```python
from build123d import *

# Parameters (mm, degrees)
BOSS_EXTRUDE1_DEPTH     = 2
SCALE1_SCALE            = 2
SKETCH6_R               = 1.5
CUT_EXTRUDE2_DEPTH      = 50.464206186
SKETCH7_W               = 25
SKETCH7_H               = 3
BOSS_EXTRUDE2_DEPTH     = 15
SKETCH8_R               = 1.5
SKETCH8_W               = 16
SKETCH8_H               = 11
CUT_EXTRUDE3_DEPTH      = 18
FILLET3_R               = 3
FILLET4_R               = 3
SKETCH10_R              = 1.5
CUT_EXTRUDE4_DEPTH      = 10
CUT_EXTRUDE5_DEPTH      = 52.533558907
CUT_EXTRUDE5_DEPTH_BACK = 52.533558907
SKETCH11_W              = 25
SKETCH11_H              = 3
CUT_EXTRUDE6_DEPTH      = 50.464206186
CUT_EXTRUDE6_DEPTH_BACK = 50.464206186


with BuildPart() as part:
    # Sketch2 → Boss-Extrude1 (new body)
    with BuildSketch(Plane(origin=(0, 0, 0), x_dir=(1, 0, 0), z_dir=(0, 1, 0))):
        with BuildLine():
            Line((-17.967387551, 9.159795774), (-20.639475337, 7.15016677))
            ThreePointArc((-20.639475337, 7.15016677), (-18.649238809, 4.17439457), (-19.346117765, 0.662896123))
            ThreePointArc((-19.346117765, 0.662896123), (-19.45411943, -1.286546543), (-18.558961711, -3.021678736))
            ThreePointArc((-18.558961711, -3.021678736), (-16.421478173, -5.190969631), (-13.78312899, -6.712078584))
            ThreePointArc((-13.78312899, -6.712078584), (-13.032173848, -6.916004841), (-12.276686285, -7.102440046))
            ThreePointArc((-12.276686285, -7.102440046), (-12.194265553, -8.245293076), (-11.737308023, -9.296052821))
            ThreePointArc((-11.737308023, -9.296052821), (-10.975506649, -9.937799505), (-10.090124565, -10.394175126))
            Line((-10.090124565, -10.394175126), (-7.391598262, -11.698651137))
            Line((-7.391598262, -11.698651137), (7.391598262, -11.698651137))
            Line((7.391598262, -11.698651137), (10.090124565, -10.394175126))
            ThreePointArc((10.090124565, -10.394175126), (10.975506649, -9.937799505), (11.737308023, -9.296052821))
            ThreePointArc((11.737308023, -9.296052821), (12.194265553, -8.245293076), (12.276686285, -7.102440046))
            ThreePointArc((12.276686285, -7.102440046), (13.032173848, -6.916004841), (13.78312899, -6.712078584))
            ThreePointArc((13.78312899, -6.712078584), (16.421478173, -5.190969631), (18.558961711, -3.021678736))
            ThreePointArc((18.558961711, -3.021678736), (19.45411943, -1.286546543), (19.346117765, 0.662896123))
            ThreePointArc((19.346117765, 0.662896123), (18.649238809, 4.17439457), (20.639475337, 7.15016677))
            Line((20.639475337, 7.15016677), (17.967387551, 9.159795774))
            ThreePointArc((17.967387551, 9.159795774), (10.858325227, 7.499674132), (4.169484372, 10.424426945))
            Line((4.169484372, 10.424426945), (2.224138848, 10.424426945))
            Line((2.224138848, 10.424426945), (0.696104526, 13.114793475))
            Line((0.696104526, 13.114793475), (0, 13.358013588))
            Line((0, 13.358013588), (-0.696104526, 13.114793475))
            Line((-0.696104526, 13.114793475), (-2.224138848, 10.424426945))
            Line((-2.224138848, 10.424426945), (-4.169484372, 10.424426945))
            ThreePointArc((-4.169484372, 10.424426945), (-10.858325227, 7.499674132), (-17.967387551, 9.159795774))
        make_face()
    extrude(amount=BOSS_EXTRUDE1_DEPTH)


with BuildPart() as part_1:
    # Scale1: scaled about (0, 1, 0.242383844)
    add(part.part.scale(SCALE1_SCALE).moved(Location((0, -1, -0.242383844))))

    # Sketch6 → Cut-Extrude2 (cut, through all)
    with BuildSketch(Plane(origin=(0, 3, 0), x_dir=(1, 0, 0), z_dir=(0, 1, 0))):
        with Locations(Location((-5.851533015, 16.28357055, 0), (0, 0, 270))):
            Circle(SKETCH6_R)
        with Locations(Location((4.151829214, 16.28357055, 0), (0, 0, 270))):
            Circle(SKETCH6_R)
    extrude(amount=-CUT_EXTRUDE2_DEPTH, mode=Mode.SUBTRACT)

    # Sketch7 → Boss-Extrude2 (add)
    with BuildSketch(Plane(origin=(0, 3, 0), x_dir=(1, 0, 0), z_dir=(0, 1, 0))):
        with Locations((0, 11.610861671)):
            Rectangle(SKETCH7_W, SKETCH7_H)
    extrude(amount=BOSS_EXTRUDE2_DEPTH)

    # Sketch8 → Cut-Extrude3 (cut)
    with BuildSketch(Plane.XY.offset(-10.110861671)):
        with Locations((-9.75, 10.917386914)):
            Circle(SKETCH8_R)
        with Locations((9.75, 10.917386914)):
            Circle(SKETCH8_R)
        with Locations((0, 10.917386914)):
            Rectangle(SKETCH8_W, SKETCH8_H)
    extrude(amount=-CUT_EXTRUDE3_DEPTH, mode=Mode.SUBTRACT)

    # Fillet3
    fillet3_edges = [part_1.edges().sort_by_distance(p)[0] for p in [
        (-12.5, 18, -11.610861671),
    ]]
    fillet(fillet3_edges, radius=FILLET3_R)

    # Fillet4
    fillet4_edges = [part_1.edges().sort_by_distance(p)[0] for p in [
        (12.5, 18, -11.610861671),
    ]]
    fillet(fillet4_edges, radius=FILLET4_R)

    # Sketch10 → Cut-Extrude4 (cut)
    with BuildSketch(Plane(origin=(0, 3, 0), x_dir=(1, 0, 0), z_dir=(0, 1, 0))):
        with Locations(Location((-0.8498519, -20.895328087, 0), (0, 0, 270))):
            Circle(SKETCH10_R)
    extrude(amount=-CUT_EXTRUDE4_DEPTH, mode=Mode.SUBTRACT)

    # Sketch11 → Cut-Extrude5 (cut, two sides: drawn at the far end of the back side and taken through both)
    with BuildSketch(Plane(origin=(0, 3, 0), x_dir=(1, 0, 0), z_dir=(0, 1, 0)).offset(-CUT_EXTRUDE5_DEPTH_BACK)):
        with Locations((0, 11.610861671)):
            Rectangle(SKETCH11_W, SKETCH11_H)
    extrude(amount=CUT_EXTRUDE5_DEPTH + CUT_EXTRUDE5_DEPTH_BACK, mode=Mode.SUBTRACT)

    # Sketch12 → Cut-Extrude6 (cut, two sides: drawn at the far end of the back side and taken through both)
    with BuildSketch(Plane(origin=(0, 3, 0), x_dir=(1, 0, 0), z_dir=(0, 1, 0)).offset(-CUT_EXTRUDE6_DEPTH_BACK)):
        with BuildLine():
            Line((-5.923543235, 0), (5.923543235, 0))
            ThreePointArc((5.923543235, 0), (6.842985975, -0.606776086), (6.646636982, -1.690749907))
            Line((6.646636982, -1.690749907), (0.723093747, -7.891658559))
            ThreePointArc((0.723093747, -7.891658559), (0, -8.200908652), (-0.723093747, -7.891658559))
            Line((-0.723093747, -7.891658559), (-6.646636982, -1.690749907))
            ThreePointArc((-6.646636982, -1.690749907), (-6.842985975, -0.606776086), (-5.923543235, 0))
        make_face()
    extrude(amount=CUT_EXTRUDE6_DEPTH + CUT_EXTRUDE6_DEPTH_BACK, mode=Mode.SUBTRACT)


solid = part_1.part
```
Read the model definition and answer for the solid it produces. Units are mm, in the model's axes. A direction names the side the tool comes from. Coordinates: 2 decimals unless noted, no trailing zeros. Order: outer loops, then holes, each group sorted by start corner. A loop starts at its lowest first (then second) coordinate and runs counter-clockwise, first axis right, second up. Notation, with made-up numbers: (49, 15) - (103, 15) arc R32 cw to (103, 48) - close; hole circle Ø5 at (26, -19). An arc over 180 degrees is marked (long way). Answer as a JSON object with one key per item and string values. Group by question number.
Item 1: A tool of negligible diameter and unlimited length cuts with its end or side. For faces 1 (the face through (-37.32, 0.97, -8.69)), 2 (the face through (0, 1, -13.111)), from which of +Z, -Z, +X, -X, +Y, -Y can it reach the whole face along a straight path? Write none if from no direction.
Item 2: Section A-A (x = -11) is taken. Give the vertices of the cut face in (y, z), plus the area to 3 significant figures.
Item 3: Section C-C (z = -9) is taken. Give the vertices of the cut face in (x, y), plus the area to 3 significant figures.
Item 4: Flat-ended cylindrical pins translate along their axes: P1, Ø2.5, axis at x = -5.85, z = -16.28, coming from the -Y side; P2, Ø4, axis at x = 4.15, z = -16.28, coming from the -Y side; P3, Ø1.2, axis at x = 6.5, y = 1, coming from the -Z side; P4, Ø2, axis at y = 1.5, z = 17.5, coming from the +X side. Find the tip coordinate at first contact, or state that the pin passes through.
Item 5: Consider probe 1 along Z at (x, y) = (-5, -0.4); probe 2 along Z at (x, y) = (8, 1.8); probe 3 along Z at (x, y) = (1, 2.6). Determine where each line is inside the solid, lowest interval first. Write a range as from..to.
Item 6: Section B-B (y = 0.85) is taken. State how many separate pieces and enclosed holes the cut face has, plus the area to 3 significant figures.
Item 7: Section D-D (x = -30.5) is taken. Give the vertices of the cut face in (y, z).
Item 8: The mould has two halves that part along Z. Classify faces 3 (the face through (32.78, 0.97, 10.19)), 4 (the face through (-6, 1, -21.091)), 5 (the face through (-0.784, 1.028, 19.397)): +Z half, -Z half, draft (parallel to the pull), parting line (faces both ways), or undercut.
Results are:
{
 "1": {"face 1": "-X, +Y, -Y", "face 2": "+Y, -Y"},
 "2": {"outline": "(-1, -19.03) - (3, -19.03) - (3, -13.11) - (-1, -13.11) - close; (-1, -10.11) - (3, -10.11) - (3, 23.15) - (-1, 23.15) - close", "area": "157 mm^2"},
 "3": {"outline": "(-37.39, -1) - (37.39, -1) - (37.39, 3) - (-37.39, 3) - close", "area": "299 mm^2"},
 "4": {"P1": "passes through", "P2": "stops at y = -1", "P3": "stops at z = -21.09", "P4": "stops at x = 24.32"},
 "5": {"probe 1": "z = -21.09..-17.52, -15.05..-13.11, -10.11..0, 3.41..23.15", "probe 2": "z = -21.09..-13.11, -10.11..23.15", "probe 3": "z = -26.61..-13.11, -10.11..0, 7.6..23.15"},
 "6": {"separate pieces": "1", "enclosed holes": "5", "area": "2,610 mm^2"},
 "7": {"outline": "(-1, -16.13) - (3, -16.13) - (3, 11.73) - (-1, 11.73) - close"},
 "8": {"face 3": "+Z half", "face 4": "-Z half", "face 5": "undercut"}
}
